Can you work these out from the drawing? Everything is in mm from the part's minimum corner. A direction names the side the tool comes from. Give positions to 0.01 mm unless a question says otherwise; leave off trailing zeros. Loops run counter-clockwise (first coordinate to the right, second up) from the corner with the lowest first, then second, coordinate; pieces in that order, holes last. Notation, with made-up numbers: (51.25, -11) -> (56.25, -11) arc R19 cw to (56.25, 15) -> close; hole circle Ø8 at (19.5, 47.5). An arc over 180 degrees is marked (long way). Write item = value, one per line. Start each with the question number.
1) On a 3-axis mill with a long thin cutter (end or side, diameter ignored), from which of +Z, -Z, +X, -X, +Y, -Y can I reach the whole of each face in a straight line? I mean the marked faces 4 and 5. Say none if no direction works.
2) I need wall thicknesses on probe 1 along Y at (x, z) = (17.5, 1.2) (1 decimal); probe 2 along X at (y, z) = (6, 1.35) (1 decimal); probe 3 along X at (y, z) = (19, 1.9) (1 decimal). Which ranges of each line are inside material? Lowest first, please. Write a range as from..to.
3) If we mould it in two halves opening along Y, with no side actions, what happens to the marked faces 1, 2 and 3? For each: +Y half, -Y half, draft (parallel to the pull), parting line (faces both ways), or undercut.
4) I'm going to push a flat-ended pin straight in: pin 1 Ø2 at (x, y) = (6.8, 7.07) entering from -Z. Where does the tip first touch, or does it pass through?
5) I want a section at A-A (y = 32.5). List the corners of the cut face in (x, z) for me (1 decimal).
6) I want a section at B-B (z = 1.5). List the corners of the cut face in (x, y) for me (1 decimal), and give its area (4 significant figures).
7) I want a section at C-C (y = 25.5). List the corners of the cut face in (x, z) for me (1 decimal).
8) I want a section at D-D (y = 12). List the corners of the cut face in (x, z) for me (1 decimal).
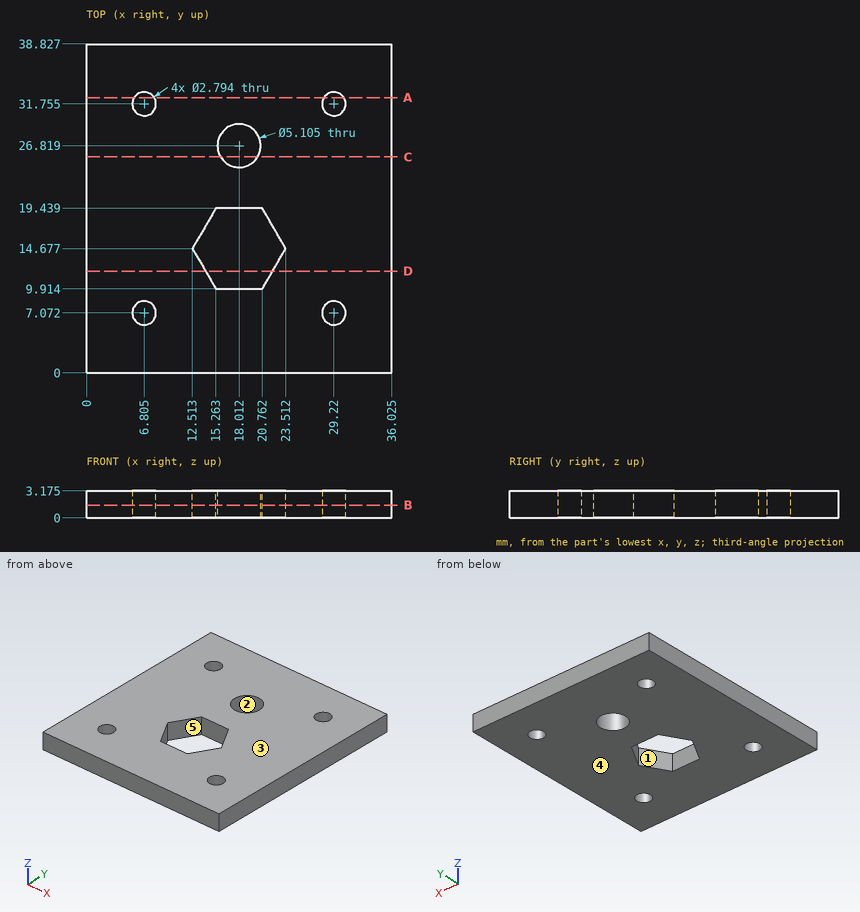
Answer list:
q1.face_4 = -Z, +X, -X, +Y, -Y
q1.face_5 = +Z, -Z
q2.probe_1 = 0..9.9, 19.4..24.3, 29.3..38.8
q2.probe_2 = 0..5.9, 7.7..28.3, 30.1..36
q2.probe_3 = 0..15, 21..36
q3.face_1 = undercut
q3.face_2 = undercut
q3.face_3 = draft
q4.pin_1 = through
q5.outline = (0, 0) -> (5.6, 0) -> (5.6, 3.2) -> (0, 3.2) -> close; (8, 0) -> (28, 0) -> (28, 3.2) -> (8, 3.2) -> close; (30.4, 0) -> (36, 0) -> (36, 3.2) -> (30.4, 3.2) -> close
q6.outline = (0, 0) -> (36, 0) -> (36, 38.8) -> (0, 38.8) -> close; hole circle Ø2.8 at (6.8, 7.1); hole circle Ø2.8 at (6.8, 31.8); hole (12.5, 14.7) -> (15.3, 9.9) -> (20.8, 9.9) -> (23.5, 14.7) -> (20.8, 19.4) -> (15.3, 19.4) -> close; hole circle Ø5.1 at (18, 26.8); hole circle Ø2.8 at (29.2, 7.1); hole circle Ø2.8 at (29.2, 31.8)
q6.area = 1,275 mm^2
q7.outline = (0, 0) -> (15.8, 0) -> (15.8, 3.2) -> (0, 3.2) -> close; (20.2, 0) -> (36, 0) -> (36, 3.2) -> (20.2, 3.2) -> close
q8.outline = (0, 0) -> (14.1, 0) -> (14.1, 3.2) -> (0, 3.2) -> close; (22, 0) -> (36, 0) -> (36, 3.2) -> (22, 3.2) -> close
